Could you check a few things on this model? Use its own coordinates, in mm. A direction names the side the tool comes from. Give positions to 0.01 mm unless a question says otherwise; leave off trailing zeros. Write each loop counter-clockwise with the first axis right and the second up, starting at its lowest first coordinate (ties: lowest second). Pieces come first, ordered by that corner, then holes. Notation, with made-up numbers: (7, 28.5) - (62, 28.5) arc R20 cw to (62, 57.5) - close; hole circle Ø2 at (23, -32). An arc over 180 degrees is marked (long way). Answer as CSV lines item,"result". Start each with the question number.
Q1. If I drill on line 1 along X through (y, z) = (1.25, 4.5); line 2 along X through (y, z) = (2, 5); line 3 along Y through (x, z) = (6, 5.5), over which ranges is the centre line in solid material (lowest first)?
Q2. Imagine slicing it at B-B on x = 2.5. List the corners of the cut face in (y, z) for me, and give its area (3 significant figures).
Q3. Will these pins go through, and if not, where does the flat tip stop? pin 1 Ø1.5 at (x, z) = (1, 6.5) entering from +Y; pin 2 Ø1 at (y, z) = (1.5, 3.5) entering from +X.
Q4. Imagine slicing it at D-D on y = 3. List the corners of the cut face in (x, z) for me, and give its area (3 significant figures).
Q5. On a 3-axis mill with a long thin cutter (end or side, diameter ignored), from which of +Z, -Z, +X, -X, +Y, -Y can I reach the whole of each face in a straight line? I mean faces 1 (the face through (6, 0, 4)), 2 (the face through (3, 1, 1.473)). Say none if no direction works.
Q6. Imagine slicing it at A-A on y = 1.75. List the corners of the cut face in (x, z) for me.
Q7. We'd pull the mould along Z, two halves only. Please class faces 3 (the face through (3.953, 3.191, 3.844)), 4 (the face through (1.473, 2, 4)), 5 (the face through (2, 2, 0)), 6 (the face through (2, 2, 7.798)): pulls with the +Z half, pulls with the -Z half, needs draft (parallel to the pull), parting line crosses it, or undercut.
Q8. Imagine slicing it at C-C on z = 3.75. List the corners of the cut face in (x, y) for me, and give its area (3 significant figures).
Autodesk Inventor part; units mm, degrees
ref_plane "YZ Plane" through (0, 0, 0) normal (1, 0, 0) x (0, 1, 0)
ref_plane "XZ Plane" through (0, 0, 0) normal (0, 1, 0) x (-1, 0, 0)
ref_plane "XY Plane" through (0, 0, 0) normal (0, 0, 1) x (1, 0, 0)
sketch "Sketch1" plane through (0, 0, 0) normal (0, 0, 1) x (1, 0, 0)
  line L0 (0, 0) -> (0, 6.4719)
  line L1 (0, 0) -> (7.7978, 0)
  line L2 (7.7978, 0) -> (0, 6.4719)
  dimension "d0" = 6.4719
  dimension "d1" = 7.7978
extrude "Extrusion1" add sketch "Sketch1" along normal blind 7.7978
shell "Shell1" thickness 1.4732 removed faces 1 at (5.1985, 0, 2.5993)
properties part number "Transparent Grey Peice" material "ABS Plastic"
Conclusion:
1,line 1,"0 to 1.47, 3.98 to 6.29"
1,line 2,"0 to 1.47, 3.08 to 5.39"
1,line 3,"0 to 1.49"
2,outline,"(0, 0) - (4.4, 0) - (4.4, 7.8) - (0, 7.8) - (0, 6.32) - (2.48, 6.32) - (2.48, 1.47) - (0, 1.47) - close"
2,area,"22.2 mm^2"
3,pin 1,"y = 6.26"
3,pin 2,"x = 6.59"
4,outline,"(0, 0) - (4.18, 0) - (4.18, 7.8) - (0, 7.8) - close; hole (1.47, 1.47) - (1.88, 1.47) - (1.88, 6.32) - (1.47, 6.32) - close"
4,area,"30.7 mm^2"
5,face 1,"+Z, -Z, +X, -X, -Y"
5,face 2,"-Y"
6,outline,"(0, 0) - (5.69, 0) - (5.69, 7.8) - (0, 7.8) - close; hole (1.47, 1.47) - (3.38, 1.47) - (3.38, 6.32) - (1.47, 6.32) - close"
7,face 3,"needs draft"
7,face 4,"undercut"
7,face 5,"pulls with the -Z half"
7,face 6,"pulls with the +Z half"
8,outline,"(0, 0) - (1.47, 0) - (1.47, 3.33) - (5.49, 0) - (7.8, 0) - (0, 6.47) - close"
8,area,"18.5 mm^2"
